from build123d import *

# Parameters (mm, degrees)
F0_W      = 1066.8
F0_H      = 1993.9
F1_DEPTH  = 101.6
F2_W      = 1028.7
F2_H      = 1955.8
F3_DEPTH  = 82.55
F4_W      = 825.5
F4_H      = 508
F5_DEPTH  = 19.051
F6_W      = 1066.8
F6_H      = 25.4
F7_DEPTH  = 50.8
F8_W      = 19.05
F8_H      = 31.75
F9_DEPTH  = 1066.801
F11_D     = 15.875
F11_DEPTH = 12.7
F11_TIP   = 4.7693311635
F13_D     = 8.4328
F13_DEPTH = 12.7
F13_TIP   = 2.5334687141
F14_W     = 50.8
F14_H     = 1955.8
F15_DEPTH = 12.7
F16_W     = 1955.8
F16_H     = 6.35
F17_DEPTH = 44.45
F18_W     = 1955.8
F18_H     = 6.35
F19_DEPTH = 44.45
F20_W     = 44.45
F20_H     = 736.6
F21_DEPTH = 12.7


with BuildPart() as f1:
    # F0 (on Top) → F1 (new body)
    with BuildSketch(Plane.XY):
        with Locations((533.4, 996.95)):
            Rectangle(F0_W, F0_H)
    extrude(amount=F1_DEPTH)

    # F2 (on face) → F3 (cut)
    with BuildSketch(Plane.XY.offset(101.6)):
        with Locations((533.4, 996.95)):
            Rectangle(F2_W, F2_H)
    extrude(amount=-F3_DEPTH, mode=Mode.SUBTRACT)

    # F4 (on face) → F5 (cut, through all)
    with BuildSketch(Plane.XY.offset(19.05)):
        with Locations((533.4, 1619.25)):
            Rectangle(F4_W, F4_H)
        with Locations((533.4, 374.65)):
            Rectangle(F4_W, F4_H)
    extrude(amount=-F5_DEPTH, mode=Mode.SUBTRACT)

    # F6 (on face) → F7 (join)
    with BuildSketch(Plane.XY.offset(101.6)):
        with Locations((533.4, 2006.6)):
            Rectangle(F6_W, F6_H)
        with Locations((533.4, -12.7)):
            Rectangle(F6_W, F6_H)
    extrude(amount=-F7_DEPTH)

    # F8 (on face) → F9 (cut, through all)
    with BuildSketch(Plane(origin=(0, 0, 0), x_dir=(0, -1, 0), z_dir=(-1, 0, 0))):
        with Locations((-2003.425, 66.675)):
            Rectangle(F8_W, F8_H)
        with Locations((9.525, 66.675)):
            Rectangle(F8_W, F8_H)
    extrude(amount=-F9_DEPTH, mode=Mode.SUBTRACT)

    # F11
    with Locations(Plane(origin=(0, 2019.3, 0), x_dir=(-1, 0, 0), z_dir=(0, 1, 0))):
        with Locations((-939.8, 76.2), (-533.4, 76.2), (-127, 76.2)):
            Hole(F11_D / 2, depth=F11_DEPTH)
            with Locations((0, 0, -(F11_DEPTH + F11_TIP / 2))):  # 118° drill point
                Cone(0, F11_D / 2, F11_TIP, mode=Mode.SUBTRACT)

    # F13
    with Locations(Plane.XZ.offset(25.4)):
        with Locations((127, 76.2), (533.4, 76.2), (939.8, 76.2)):
            Hole(F13_D / 2, depth=F13_DEPTH)
            with Locations((0, 0, -(F13_DEPTH + F13_TIP / 2))):  # 118° drill point
                Cone(0, F13_D / 2, F13_TIP, mode=Mode.SUBTRACT)

    # F14 (on face) → F15 (join)
    with BuildSketch(Plane.XY.offset(19.05)):
        with Locations((95.25, 996.95)):
            Rectangle(F14_W, F14_H)
        with Locations((971.55, 996.95)):
            Rectangle(F14_W, F14_H)
    extrude(amount=F15_DEPTH)

    # F16 (on face) → F17 (cut)
    with BuildSketch(Plane(origin=(946.15, 0, 0), x_dir=(0, -1, 0), z_dir=(-1, 0, 0))):
        with Locations((-996.95, 22.225)):
            Rectangle(F16_W, F16_H)
    extrude(amount=-F17_DEPTH, mode=Mode.SUBTRACT)

    # F18 (on face) → F19 (cut)
    with BuildSketch(Plane.YZ.offset(120.65)):
        with Locations((996.95, 22.225)):
            Rectangle(F18_W, F18_H)
    extrude(amount=-F19_DEPTH, mode=Mode.SUBTRACT)

    # F20 (on face) → F21 (cut, through all)
    with BuildSketch(Plane.XY.offset(31.75)):
        with Locations((968.375, 996.95)):
            Rectangle(F20_W, F20_H)
        with Locations((98.425, 996.95)):
            Rectangle(F20_W, F20_H)
    extrude(amount=-F21_DEPTH, mode=Mode.SUBTRACT)


solid = f1.part
Design review of the part built by this model. Coordinates are the model's own, in mm. A direction names the side the tool comes from. Coordinates: 2 decimals unless noted, no trailing zeros. Order: outer loops, then holes, each group sorted by start corner. A loop starts at its lowest first (then second) coordinate and runs counter-clockwise, first axis right, second up. Notation, with made-up numbers: (22, 0) -> (68, 0) arc R35 ccw to (68, 36) -> close; hole circle Ø11 at (80, -17). An arc over 180 degrees is marked (long way). One line per item, written item: value.
1) Machinability: for faces 1 (the face through (99, 320, 25.4)), 2 (the face through (994, 1011, 31.75)), 3 (the face through (526, -25.4, 77)), 4 (the face through (526, 1232, 0)), 5 (the face through (526, 1993.9, 41)), which of the approach directions +Z, -Z, +X, -X, +Y, -Y give a long, thin tool a straight path to every point of the face, cutting with its end or side? Answer none if there is none.
Output values:
face 1: none
face 2: +Z
face 3: +Z, -Z, +X, -X, -Y
face 4: -Z, +X, -X, +Y, -Y
face 5: -Z, +X, -X
2) Draft analysis for pull direction Y (two halves, no side actions). For faces 6 (the face through (1047.75, 983, 61)), 7 (the face through (526, 2019.3, 82)), 8 (the face through (17, 1002, 101.6)), state which applies: +Y half, -Y half, draft (parallel to the pull), parting line (faces both ways), or undercut.
Output values:
face 6: undercut
face 7: +Y half
face 8: draft
3) Clearance check with flat-ended pins moving along their axes: P1, Ø21, axis at x = 701, z = 5.5, coming from the +Y side; P2, Ø3, axis at x = 854.5, y = 788, coming from the +Z side; P3, Ø1.9, axis at x = 95.5, z = 29.5, coming from the -Y side. State where each tip first meets the part, or that it passes through.
Output values:
P1: stops at y = 1993.9
P2: stops at z = 19.05
P3: stops at y = 0
4) We need section D-D, the plane y = 971. Give the boundary of the cut face in (x, z), then the cut area to 3 significant figures.
Output values:
outline: (0, 0) -> (1066.8, 0) -> (1066.8, 101.6) -> (1047.75, 101.6) -> (1047.75, 19.05) -> (996.95, 19.05) -> (996.95, 31.75) -> (990.6, 31.75) -> (990.6, 19.05) -> (76.2, 19.05) -> (76.2, 31.75) -> (69.85, 31.75) -> (69.85, 19.05) -> (19.05, 19.05) -> (19.05, 101.6) -> (0, 101.6) -> close
area: 23,600 mm2
5) We need section C-C, the plane x = 98.5. Give the boundary of the cut face in (y, z), then the cut area to 3 significant figures.
Output values:
outline: (-25.4, 50.8) -> (-19.05, 50.8) -> (-19.05, 82.55) -> (0, 82.55) -> (0, 0) -> (1993.9, 0) -> (1993.9, 82.55) -> (2012.95, 82.55) -> (2012.95, 50.8) -> (2019.3, 50.8) -> (2019.3, 101.6) -> (1974.85, 101.6) -> (1974.85, 31.75) -> (1365.25, 31.75) -> (1365.25, 25.4) -> (1974.85, 25.4) -> (1974.85, 19.05) -> (19.05, 19.05) -> (19.05, 25.4) -> (628.65, 25.4) -> (628.65, 31.75) -> (19.05, 31.75) -> (19.05, 101.6) -> (-25.4, 101.6) -> close
area: 50,200 mm2
6) We need section B-B, the plane y = 376.5. Give the boundary of the cut face in (x, z), then the cut area to 3 significant figures.
Output values:
outline: (0, 0) -> (120.65, 0) -> (120.65, 19.05) -> (76.2, 19.05) -> (76.2, 25.4) -> (120.65, 25.4) -> (120.65, 31.75) -> (69.85, 31.75) -> (69.85, 19.05) -> (19.05, 19.05) -> (19.05, 101.6) -> (0, 101.6) -> close; (946.15, 0) -> (1066.8, 0) -> (1066.8, 101.6) -> (1047.75, 101.6) -> (1047.75, 19.05) -> (996.95, 19.05) -> (996.95, 31.75) -> (946.15, 31.75) -> (946.15, 25.4) -> (990.6, 25.4) -> (990.6, 19.05) -> (946.15, 19.05) -> close
area: 8,470 mm2
7) To check wall thickness, follow probe 1 along Y at (x, z) = (213, 61); probe 2 along X at (y, z) = (2013.75, 76.2); probe 3 along X at (y, z) = (988, 26). State the ranges of each line that lie inside material, in increasing order. Write a range as [from, to].
Output values:
probe 1: y = [-25.4, -19.05], [0, 19.05], [1974.85, 1993.9], [2012.95, 2019.3]
probe 2: x = [0, 119.06], [134.94, 525.46], [541.34, 931.86], [947.74, 1066.8]
probe 3: x = [0, 19.05], [69.85, 76.2], [990.6, 996.95], [1047.75, 1066.8]
8) We need section A-A, the plane x = 380.5. Give the boundary of the cut face in (y, z).
Output values:
outline: (-25.4, 50.8) -> (-19.05, 50.8) -> (-19.05, 82.55) -> (0, 82.55) -> (0, 0) -> (120.65, 0) -> (120.65, 19.05) -> (19.05, 19.05) -> (19.05, 101.6) -> (-25.4, 101.6) -> close; (628.65, 0) -> (1365.25, 0) -> (1365.25, 19.05) -> (628.65, 19.05) -> close; (1873.25, 0) -> (1993.9, 0) -> (1993.9, 82.55) -> (2012.95, 82.55) -> (2012.95, 50.8) -> (2019.3, 50.8) -> (2019.3, 101.6) -> (1974.85, 101.6) -> (1974.85, 19.05) -> (1873.25, 19.05) -> close
